from build123d import *

# Parameters (mm, degrees)
SKETCH1_R               = 3.175
BOSS_EXTRUDE1_DEPTH     = 38.1
SKETCH2_R               = 0.524148551
CUT_EXTRUDE1_DEPTH      = 0.508
CUT_EXTRUDE2_DEPTH      = 74.375236584
CUT_EXTRUDE2_DEPTH_BACK = 74.375236584
SKETCH4_W               = 15.24
SKETCH4_H               = 29.21
CHAMFER1_SIZE           = 3.76570486
CHAMFER1_SIZE_2         = 2.54
FILLET1_R               = 1.27


with BuildPart() as part:
    # Sketch1 → Boss-Extrude1 (new body)
    with BuildSketch(Plane.XY):
        with BuildLine():
            ThreePointArc((3.431040036, -1.656521739), (1.656521739, 3.431040036), (-3.431040036, 1.656521739))
            ThreePointArc((-3.431040036, 1.656521739), (-31.969026999, -12.060345778), (-51.704640275, 12.7))
            ThreePointArc((-51.704640275, 12.7), (-55.514640275, 16.51), (-59.324640275, 12.7))
            ThreePointArc((-59.324640275, 12.7), (-33.668343017, -19.488449511), (3.431040036, -1.656521739))
        make_face()
        with Locations(Location((-26.304640275, -16.51, 0), (0, 0, 180))):
            Circle(SKETCH1_R, mode=Mode.SUBTRACT)
    extrude(amount=BOSS_EXTRUDE1_DEPTH)

    # Sketch2 → Cut-Extrude1 (cut)
    with BuildSketch(Plane.XY.offset(38.1)):
        Circle(SKETCH2_R)
    cut_extrude1 = extrude(amount=-CUT_EXTRUDE1_DEPTH, mode=Mode.SUBTRACT)

    # Mirror1: Cut-Extrude1 across plane
    add(cut_extrude1.mirror(Plane.XY.offset(19.05)), mode=Mode.SUBTRACT)

    # Sketch4 → Cut-Extrude2 (cut, two sides: drawn at the far end of the back side and taken through both)
    with BuildSketch(Plane(origin=(0, 0, 0), x_dir=(0, 0, -1), z_dir=(1, 0, 0)).offset(-CUT_EXTRUDE2_DEPTH_BACK)):
        with Locations((-19.05, 1.905)):
            Rectangle(SKETCH4_W, SKETCH4_H)
    extrude(amount=CUT_EXTRUDE2_DEPTH + CUT_EXTRUDE2_DEPTH_BACK, mode=Mode.SUBTRACT)

    # Chamfer1
    # the kernel refuses this chamfer: 3.76570486, 2.54 mm, written as the material it takes off along each edge
    with BuildSketch(Plane(origin=(-26.304640275, 12.7, 26.67), x_dir=(0.9005354424873034, -0.43478260869565205, 0), z_dir=(0.43478260869565205, 0.9005354424873034, 0))) as chamfer1_piece_1_section:
        Polygon((25.4, -CHAMFER1_SIZE), (25.4 + CHAMFER1_SIZE_2, 0), (25.4, 0), align=None)
    chamfer1_piece_1 = revolve(axis=Axis((-26.304640275, 12.7, 26.67), (0, 0, -1)), revolution_arc=64.228538259, mode=Mode.PRIVATE)
    chamfer1_piece_1 = split(chamfer1_piece_1, bisect_by=Plane(origin=(-26.304640275, -12.7, 26.67), z_dir=(0, 1, 0)), keep=Keep.TOP, mode=Mode.PRIVATE)
    add(chamfer1_piece_1, mode=Mode.SUBTRACT)
    with BuildSketch(Plane(origin=(-26.304640275, 12.7, 26.67), x_dir=(0.9005354424873037, -0.43478260869565155, 0), z_dir=(0.43478260869565155, 0.9005354424873037, 0))) as chamfer1_piece_2_section:
        Polygon((33.02, -CHAMFER1_SIZE), (33.02 - CHAMFER1_SIZE_2, 0), (33.02, 0), align=None)
    chamfer1_piece_2 = revolve(axis=Axis((-26.304640275, 12.7, 26.67), (0, 0, -1)), revolution_arc=41.395045941, mode=Mode.PRIVATE)
    chamfer1_piece_2 = split(chamfer1_piece_2, bisect_by=Plane(origin=(-26.304640275, -12.7, 26.67), z_dir=(0, 1, 0)), keep=Keep.TOP, mode=Mode.PRIVATE)
    add(chamfer1_piece_2, mode=Mode.SUBTRACT)
    with BuildSketch(Plane(origin=(0, 0, 26.67), x_dir=(-0.9005354424873006, 0.4347826086956581, 0), z_dir=(-0.4347826086956581, -0.9005354424873006, 0))) as chamfer1_piece_3:
        Polygon((3.81, -CHAMFER1_SIZE), (3.81 - CHAMFER1_SIZE_2, 0), (3.81, 0), align=None)
    revolve(axis=Axis((0, 0, 26.67), (0, 0, -1)), revolution_arc=180, mode=Mode.SUBTRACT)
    with BuildSketch(Plane(origin=(-26.304640275, 12.7, 26.67), x_dir=(0, -1, 0), z_dir=(1, 0, 0))) as chamfer1_piece_4_section:
        Polygon((25.4 + CHAMFER1_SIZE_2, 0), (25.4, -CHAMFER1_SIZE), (25.4, 0), align=None)
    chamfer1_piece_4 = revolve(axis=Axis((-26.304640275, 12.7, 26.67), (0, 0, -1)), revolution_arc=90, mode=Mode.PRIVATE)
    chamfer1_piece_4 = split(chamfer1_piece_4, bisect_by=Plane(origin=(-26.304640275, -12.7, 26.67), z_dir=(0, 1, 0)), keep=Keep.TOP, mode=Mode.PRIVATE)
    add(chamfer1_piece_4, mode=Mode.SUBTRACT)
    with BuildSketch(Plane(origin=(-55.514640275, 12.7, 26.67), x_dir=(1, 0, 0), z_dir=(0, -1, 0))) as chamfer1_piece_5:
        Polygon((3.81 - CHAMFER1_SIZE_2, 0), (3.81, CHAMFER1_SIZE), (3.81, 0), align=None)
    revolve(axis=Axis((-55.514640275, 12.7, 26.67), (0, 0, 1)), revolution_arc=180, mode=Mode.SUBTRACT)
    with BuildSketch(Plane(origin=(-26.304640275, 12.7, 26.67), x_dir=(-0.38802844135428005, -0.9216473993345654, 0), z_dir=(0.9216473993345654, -0.38802844135428005, 0))) as chamfer1_piece_6_section:
        Polygon((33.02, -CHAMFER1_SIZE), (33.02 - CHAMFER1_SIZE_2, 0), (33.02, 0), align=None)
    chamfer1_piece_6 = revolve(axis=Axis((-26.304640275, 12.7, 26.67), (0, 0, -1)), revolution_arc=67.168121234, mode=Mode.PRIVATE)
    chamfer1_piece_6 = split(chamfer1_piece_6, bisect_by=Plane(origin=(-26.304640275, -12.7, 26.67), z_dir=(0, 1, 0)), keep=Keep.TOP, mode=Mode.PRIVATE)
    add(chamfer1_piece_6, mode=Mode.SUBTRACT)
    with BuildSketch(Plane(origin=(-26.304640275, 12.7, 11.43), x_dir=(0.9005354424873034, -0.43478260869565205, 0), z_dir=(0.43478260869565205, 0.9005354424873034, 0))) as chamfer1_piece_7_section:
        Polygon((25.4, CHAMFER1_SIZE_2), (25.4 + CHAMFER1_SIZE, 0), (25.4, 0), align=None)
    chamfer1_piece_7 = revolve(axis=Axis((-26.304640275, 12.7, 11.43), (0, 0, -1)), revolution_arc=64.228538259, mode=Mode.PRIVATE)
    chamfer1_piece_7 = split(chamfer1_piece_7, bisect_by=Plane(origin=(-26.304640275, -12.7, 11.43), z_dir=(0, 1, 0)), keep=Keep.TOP, mode=Mode.PRIVATE)
    add(chamfer1_piece_7, mode=Mode.SUBTRACT)
    with BuildSketch(Plane(origin=(-26.304640275, 12.7, 11.43), x_dir=(0, -1, 0), z_dir=(1, 0, 0))) as chamfer1_piece_8_section:
        Polygon((25.4, CHAMFER1_SIZE_2), (25.4 + CHAMFER1_SIZE, 0), (25.4, 0), align=None)
    chamfer1_piece_8 = revolve(axis=Axis((-26.304640275, 12.7, 11.43), (0, 0, -1)), revolution_arc=90, mode=Mode.PRIVATE)
    chamfer1_piece_8 = split(chamfer1_piece_8, bisect_by=Plane(origin=(-26.304640275, -12.7, 11.43), z_dir=(0, 1, 0)), keep=Keep.TOP, mode=Mode.PRIVATE)
    add(chamfer1_piece_8, mode=Mode.SUBTRACT)
    with BuildSketch(Plane(origin=(-26.304640275, 12.7, 11.43), x_dir=(-0.38802844135427855, -0.9216473993345662, 0), z_dir=(0.9216473993345662, -0.38802844135427855, 0))) as chamfer1_piece_9_section:
        Polygon((33.02, CHAMFER1_SIZE_2), (33.02 - CHAMFER1_SIZE, 0), (33.02, 0), align=None)
    chamfer1_piece_9 = revolve(axis=Axis((-26.304640275, 12.7, 11.43), (0, 0, -1)), revolution_arc=67.168121234, mode=Mode.PRIVATE)
    chamfer1_piece_9 = split(chamfer1_piece_9, bisect_by=Plane(origin=(-26.304640275, -12.7, 11.43), z_dir=(0, 1, 0)), keep=Keep.TOP, mode=Mode.PRIVATE)
    add(chamfer1_piece_9, mode=Mode.SUBTRACT)
    with BuildSketch(Plane(origin=(-26.304640275, 12.7, 11.43), x_dir=(0.9005354424873037, -0.43478260869565155, 0), z_dir=(0.43478260869565155, 0.9005354424873037, 0))) as chamfer1_piece_10_section:
        Polygon((33.02, CHAMFER1_SIZE_2), (33.02 - CHAMFER1_SIZE, 0), (33.02, 0), align=None)
    chamfer1_piece_10 = revolve(axis=Axis((-26.304640275, 12.7, 11.43), (0, 0, -1)), revolution_arc=41.395045941, mode=Mode.PRIVATE)
    chamfer1_piece_10 = split(chamfer1_piece_10, bisect_by=Plane(origin=(-26.304640275, -12.7, 11.43), z_dir=(0, 1, 0)), keep=Keep.TOP, mode=Mode.PRIVATE)
    add(chamfer1_piece_10, mode=Mode.SUBTRACT)
    with BuildSketch(Plane(origin=(-55.514640275, 12.7, 11.43), x_dir=(1, 0, 0), z_dir=(0, -1, 0))) as chamfer1_piece_11:
        Polygon((3.81, -CHAMFER1_SIZE_2), (3.81 - CHAMFER1_SIZE, 0), (3.81, 0), align=None)
    revolve(axis=Axis((-55.514640275, 12.7, 11.43), (0, 0, 1)), revolution_arc=180, mode=Mode.SUBTRACT)
    with BuildSketch(Plane(origin=(0, 0, 11.43), x_dir=(-0.9005354424873006, 0.4347826086956581, 0), z_dir=(-0.4347826086956581, -0.9005354424873006, 0))) as chamfer1_piece_12:
        Polygon((3.81 - CHAMFER1_SIZE, 0), (3.81, CHAMFER1_SIZE_2), (3.81, 0), align=None)
    revolve(axis=Axis((0, 0, 11.43), (0, 0, -1)), revolution_arc=180, mode=Mode.SUBTRACT)

    # Fillet1
    fillet1_edges = [part.edges().sort_by_distance(p)[0] for p in [
        (-5.205815663, -12.7, 19.66285243),
        (-47.403464887, -12.7, 19.66285243),
    ]]
    fillet(fillet1_edges, radius=FILLET1_R)


solid = part.part
Verification items for the finished model (mm, model axes). A direction names the side the tool comes from. Coordinates: 2 decimals unless noted, no trailing zeros. Order: outer loops, then holes, each group sorted by start corner. A loop starts at its lowest first (then second) coordinate and runs counter-clockwise, first axis right, second up.
1. Set-up check for faces 4 (the face through (-44.756, -13.633, 19.512)), 5 (the face through (-7.853, -13.633, 19.512)), 6 (the face through (-5, -7, 26.67)), 7 (the face through (-29.333, -17.464, 18.783)): record each of +Z, -Z, +X, -X, +Y, -Y from which the full face is reachable in a straight line by a thin tool's end or side.
Results found:
face 4: -X
face 5: +X
face 6: +X, -X, +Y
face 7: +Z, -Z
2. Sectioned sample at A-A, the plane y = -16.51. Record the cut outline in (x, z).
Results found:
outline: (-41.7, 0) - (-29.48, 0) - (-29.48, 38.1) - (-41.7, 38.1) - close; (-23.13, 0) - (-10.91, 0) - (-10.91, 38.1) - (-23.13, 38.1) - close
3. Scan lines: line 1 (X direction, y = -1, z = 28); line 2 (X direction, y = -14, z = 32.5); line 3 (Y direction, x = -27.5, z = 14). Record each from-to range of solid material in increasing order.
Results found:
line 1: x = -54.53 to -49.62, -2.99 to 1.92
line 2: x = -45.73 to -28.25, -24.36 to -6.88
line 3: y = -20.3 to -19.45, -13.57 to -12.7
4. Sectioned sample at B-B, the plane z = 18. Record the cut outline in (x, y) (3 decimals).
Results found:
outline: (-44.221, -15.037) arc R33.02 ccw to (-8.388, -15.037) arc R1.27 ccw to (-9.078, -12.7) - (-43.532, -12.7) arc R1.27 ccw to start; hole circle Ø6.35 at (-26.305, -16.51)
5. Go/stop test with flat-tipped pins: pin 1 Ø20.5 at (x, y) = (-47, 7) entering from -Z; pin 2 Ø6 at (y, z) = (1, 14) entering from +X; pin 3 Ø10 at (y, z) = (-10.5, 14) entering from -X; pin 4 Ø1.5 at (x, z) = (-37.5, 25) entering from +Y. Record where each tip stops, or that it passes through.
Results found:
pin 1: stops at z = 0
pin 2: stops at x = 0.48
pin 3: stops at x = -50.59
pin 4: stops at y = -12.7
6. Release check for a two-part mould opening along Z. For faces 1 (the face through (-55.43, 16.51, 34.21)), 2 (the face through (-30, -13, 38.1)), 3 (the face through (-26, -12.7, 20)) record: +Z half, -Z half, draft (parallel to the pull), parting line (faces both ways), or undercut.
Results found:
face 1: draft
face 2: +Z half
face 3: undercut
7. Sectioned sample at C-C, the plane y = -3.5. Give the number of separate pieces and of enclosed holes in the cut face, and give its area (3 significant figures).
Results found:
separate pieces: 4
enclosed holes: 0
area: 375 mm2
